The model under review builds one solid part; all positions refer to its coordinate system, in mm. Round coordinates to 2 decimals unless told otherwise and drop trailing zeros. Order: outer loops, then holes, each group sorted by start corner. A loop starts at its lowest first (then second) coordinate and runs counter-clockwise, first axis right, second up. Notation, with made-up numbers: (-19, -0.75) - (21, -0.75) arc R32 ccw to (21, 29.25) - close; hole circle Ø6 at (85, -6). An arc over 180 degrees is marked (long way). One line per question, with ' | ' between items. Start each with the question number.
Item 1: Add section C-C on z = 10.5. State the section outline as (x, y) points, and give its area (3 significant figures).
Item 2: Insertion check: pin 1 Ø6 at (x, z) = (-4, 3.5) entering from -Y; pin 2 Ø3.5 at (x, y) = (0, 0) entering from -Z; pin 3 Ø2 at (y, z) = (-2.5, 11) entering from -X; pin 4 Ø3 at (y, z) = (-4, 5) entering from -X. Each pin has a flat end and moves straight along its axis. Give the tip position at first contact, or say it passes through.
Item 3: Add section A-A on y = 0. State the section outline as (x, z) points, and give its area (3 significant figures).
Item 4: For L1, parallel to Z at x = 5.25, y = 3.5; L2, parallel to Y at x = 0, z = 5.25; L3, parallel to X at y = 1, z = 8, list the stretches that pass through material, from the lowest coordinate up. Write a range as [from, to].
Item 5: Draft analysis for pull direction Z (two halves, no side actions). For faces 1 (the face through (0.881, 3.967, 6.332)), 2 (the face through (0.2, -1.51, 6.44)), 3 (the face through (1.3, 1.3, 12.7)), state which applies: +Z half, -Z half, draft (parallel to the pull), parting line (faces both ways), or undercut.
from build123d import *

# Parameters (mm, degrees)
FILLET1_R = 2.54


with BuildPart() as part:
    # Sketch2 → Revolve1 (revolve)
    with BuildSketch(Plane.YZ, mode=Mode.PRIVATE) as revolve1_sk:
        Polygon((6.35, 0), (1.524, 0), (1.524, 12.7), (6.35, 12.7), (6.35, 10.16), (4.064, 10.16), (4.064, 2.54), (6.35, 2.54), align=None)
    revolve(revolve1_sk.sketch.rotate(Axis((0, 0, 0), (0, 0, 1)), 90), axis=Axis((0, 0, 0), (0, 0, 1)))

    # Fillet1
    # the kernel refuses this fillet: 2.54 mm, written as the material it adds along each edge
    with BuildSketch(Plane(origin=(0, 0, 10.16), x_dir=(-1, 0, 0), z_dir=(0, 1, 0))) as fillet1_piece_1:
        with BuildLine():
            CenterArc((6.604, -2.52726809), FILLET1_R, 95.739170477, 84.260829523)
            Line((4.064, -2.52726809), (4.0132, -2.52726809))
            Line((4.0132, -2.52726809), (4.0132, 0))
            Line((4.0132, 0), (4.064, 0.0508))
            ThreePointArc((4.064, 0.0508), (5.207, 0.0508), (6.34492, 0.050545362))
            Line((6.34492, 0.050545362), (6.35, 0))
        make_face()
    revolve(axis=Axis((0, 0, 10.16), (0, 0, 1)))
    with BuildSketch(Plane(origin=(0, 0, 2.54), x_dir=(-1, 0, 0), z_dir=(0, 1, 0))) as fillet1_piece_2:
        with BuildLine():
            CenterArc((6.604, 2.52726809), FILLET1_R, 180, 84.260829523)
            Line((6.35, 0), (6.34492, -0.050545362))
            ThreePointArc((6.34492, -0.050545362), (5.207, -0.0508), (4.064, -0.0508))
            Line((4.064, -0.0508), (4.0132, 0))
            Line((4.0132, 0), (4.0132, 2.52726809))
            Line((4.0132, 2.52726809), (4.064, 2.52726809))
        make_face()
    revolve(axis=Axis((0, 0, 2.54), (0, 0, 1)))


solid = part.part
Determined:
1) outline: circle Ø12.7 at (0, 0); hole circle Ø3.05 at (0, 0) | area: 119 mm2
2) pin 1: y = -6.24 | pin 2: z = 0 | pin 3: x = -6.17 | pin 4: x = -3.22
3) outline: (-6.35, 0) - (-1.52, 0) - (-1.52, 12.7) - (-6.35, 12.7) - (-6.35, 10.16) arc R2.54 cw to (-4.06, 7.63) - (-4.06, 5.07) arc R2.54 cw to (-6.35, 2.54) - close; (1.52, 0) - (6.35, 0) - (6.35, 2.54) arc R2.54 cw to (4.06, 5.07) - (4.06, 7.63) arc R2.54 cw to (6.35, 10.16) - (6.35, 12.7) - (1.52, 12.7) - close | area: 93.2 mm2
4) L1: [0, 2.54], [10.16, 12.7] | L2: [-4.06, -1.52], [1.52, 4.06] | L3: [-3.97, -1.15], [1.15, 3.97]
5) face 1: undercut | face 2: draft | face 3: +Z half
